from build123d import *

# Parameters (mm, degrees)
SKETCH1_R           = 2.159
SKETCH1_R_2         = 3.81
BOSS_EXTRUDE1_DEPTH = 1.5875
FILLET1_R           = 2.54
SKETCH2_W           = 5.08
SKETCH2_H           = 15.875
SKETCH2_W_2         = 2.54
SKETCH2_H_2         = 3.81
CUT_EXTRUDE1_DEPTH  = 1.5875
FILLET2_START       = -1
FILLET2_DEPTH       = 4
FILLET2_2_DEPTH     = 1.5875


with BuildPart() as part:
    # Sketch1 → Boss-Extrude1 (new body)
    with BuildSketch(Plane.XY):
        with BuildLine():
            Line((0, 38.1), (0, 0))
            Line((0, 0), (92.075, 0))
            Line((92.075, 0), (92.075, 38.1))
            ThreePointArc((92.075, 38.1), (81.75625, 48.41875), (71.4375, 38.1))
            Line((71.4375, 38.1), (71.4375, 9.271))
            Line((71.4375, 9.271), (20.6375, 9.271))
            Line((20.6375, 9.271), (20.6375, 38.1))
            ThreePointArc((20.6375, 38.1), (10.31875, 48.41875), (0, 38.1))
        make_face()
        with Locations((22.5425, 4.6355)):
            Circle(SKETCH1_R, mode=Mode.SUBTRACT)
        with Locations((69.5325, 4.6355)):
            Circle(SKETCH1_R, mode=Mode.SUBTRACT)
        with Locations((11.1125, 38.1)):
            Circle(SKETCH1_R_2, mode=Mode.SUBTRACT)
        with Locations((80.9625, 38.1)):
            Circle(SKETCH1_R_2, mode=Mode.SUBTRACT)
    extrude(amount=BOSS_EXTRUDE1_DEPTH)

    # Fillet1
    fillet1_edges = [part.edges().sort_by_distance(p)[0] for p in [
        (92.075, 0, 0.79375),
        (0, 0, 0.79375),
    ]]
    fillet(fillet1_edges, radius=FILLET1_R)

    # Sketch2 → Cut-Extrude1 (cut)
    with BuildSketch(Plane.XY.offset(1.5875)):
        with Locations((89.535, 22.2885)):
            Rectangle(SKETCH2_W, SKETCH2_H)
        with Locations((2.54, 22.2885)):
            Rectangle(SKETCH2_W, SKETCH2_H)
        with Locations((18.0975, 25.4)):
            Rectangle(SKETCH2_W_2, SKETCH2_H_2)
        with Locations((73.9775, 25.4)):
            Rectangle(SKETCH2_W_2, SKETCH2_H_2)
    extrude(amount=-CUT_EXTRUDE1_DEPTH, mode=Mode.SUBTRACT)

    # Fillet2: read off the stored shape, not the designer's step
    # Fillet2 outline → Fillet2 (cut)
    with BuildSketch(Plane.XY.offset(FILLET2_START)):
        with BuildLine():
            Line((92.075, 14.351), (89.535, 14.351))
            ThreePointArc((89.535, 14.351), (91.331051224, 13.607051224), (92.075, 11.811))
            Line((92.075, 11.811), (92.075, 14.351))
        make_face()
        with BuildLine():
            ThreePointArc((92.075, 32.766), (91.331051224, 30.969948776), (89.535, 30.226))
            Line((89.535, 30.226), (92.075, 30.226))
            Line((92.075, 30.226), (92.075, 32.766))
        make_face()
        with BuildLine():
            Line((0, 30.226), (2.54, 30.226))
            ThreePointArc((2.54, 30.226), (0.743948776, 30.969948776), (0, 32.766))
            Line((0, 32.766), (0, 30.226))
        make_face()
        with BuildLine():
            ThreePointArc((0, 11.811), (0.743948776, 13.607051224), (2.54, 14.351))
            Line((2.54, 14.351), (0, 14.351))
            Line((0, 14.351), (0, 11.811))
        make_face()
    extrude(amount=FILLET2_DEPTH, mode=Mode.SUBTRACT)

    # Fillet2 2 outline → Fillet2 2 (add)
    with BuildSketch(Plane.XY):
        with BuildLine():
            ThreePointArc((89.535, 14.351), (87.738948776, 15.094948776), (86.995, 16.891))
            Line((86.995, 16.891), (86.995, 14.351))
            Line((86.995, 14.351), (89.535, 14.351))
        make_face()
        with BuildLine():
            ThreePointArc((86.995, 27.686), (87.738948776, 29.482051224), (89.535, 30.226))
            Line((89.535, 30.226), (86.995, 30.226))
            Line((86.995, 30.226), (86.995, 27.686))
        make_face()
        with BuildLine():
            ThreePointArc((2.54, 30.226), (4.336051224, 29.482051224), (5.08, 27.686))
            Line((5.08, 27.686), (5.08, 30.226))
            Line((5.08, 30.226), (2.54, 30.226))
        make_face()
        with BuildLine():
            ThreePointArc((5.08, 16.891), (4.336051224, 15.094948776), (2.54, 14.351))
            Line((2.54, 14.351), (5.08, 14.351))
            Line((5.08, 14.351), (5.08, 16.891))
        make_face()
    extrude(amount=FILLET2_2_DEPTH)


solid = part.part
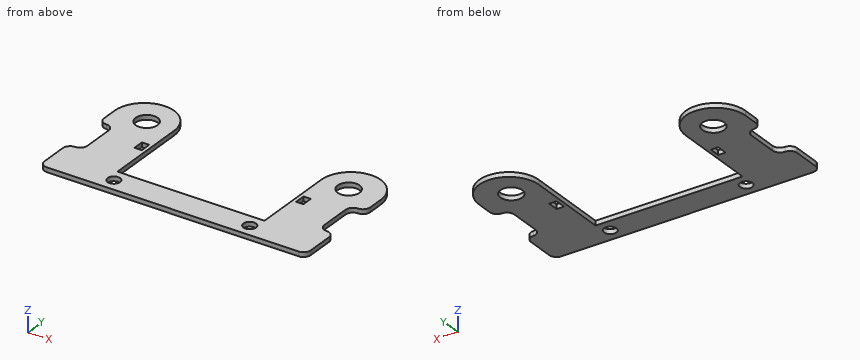
Verification items for the finished model (mm, model axes). Coordinates: 2 decimals unless noted, no trailing zeros. Order: outer loops, then holes, each group sorted by start corner. A loop starts at its lowest first (then second) coordinate and runs counter-clockwise, first axis right, second up. Notation, with made-up numbers: M 17.25,84.5 L 63.25,84.5 A29 cw 63.25,105.5 Z; hole C -22,38.25 d10. An arc over 180 degrees is marked long. One line per item, written item: value. Start each with the question number.
Item 1: Scan lines: probe 1 along X at (y, z) = (24, 0.75) (1 decimal); probe 2 along X at (y, z) = (4.5, 1.5) (3 decimals); probe 3 along X at (y, z) = (6.5, 0.25) (3 decimals). Record each from-to range of solid material in increasing order.
Item 2: Sectioned sample at C-C (z = 1.25). Count the separate pieces of the cut face and the enclosed holes in it, then the cut area to 3 significant figures.
Item 3: Sectioned sample at A-A (y = 18.5). Enter the section's corners in (x, z) (1 decimal), then the cut area to 3 significant figures.
Item 4: Sectioned sample at B-B (y = 3.5). Enter the section's corners in (x, z) (1 decimal), then the cut area to 3 significant figures.
Item 5: Gauge pin test, flat ends, axial feed: pin 1 (0.8 mm diameter, centred on y = 28, z = 1, fed in from -X); pin 2 (0.5 mm diameter, centred on y = 25, z = 1, fed in from -X); pin 3 (0.8 mm diameter, centred on y = 26, z = 1, fed in from +X) (3 decimals). Record the tip position at first contact, or that the pin passes through.
Item 6: Sectioned sample at D-D (y = 35.5). Enter the section's corners in (x, z) (1 decimal), then the cut area to 3 significant figures.
Conclusion:
1. probe 1: x = 5.1 to 16.8, 19.4 to 20.6, 71.4 to 72.7, 75.2 to 87
1. probe 2: x = 0 to 20.388, 24.697 to 67.378, 71.687 to 92.075
1. probe 3: x = 0 to 21.454, 23.631 to 68.444, 70.621 to 92.075
2. separate pieces: 1
2. enclosed holes: 6
2. area: 2,070 mm^2
3. outline: M 5.1,0 L 20.6,0 L 20.6,1.6 L 5.1,1.6 Z; M 71.4,0 L 87,0 L 87,1.6 L 71.4,1.6 Z
3. area: 49.4 mm^2
4. outline: M 0,0 L 20.7,0 L 20.7,1.6 L 0,1.6 Z; M 24.4,0 L 67.7,0 L 67.7,1.6 L 24.4,1.6 Z; M 71.4,0 L 92.1,0 L 92.1,1.6 L 71.4,1.6 Z
4. area: 135 mm^2
5. pin 1: stops at x = 4.98
5. pin 2: stops at x = 5.08
5. pin 3: stops at x = 86.995
6. outline: M 0,0 L 8.3,0 L 8.3,1.6 L 0,1.6 Z; M 13.9,0 L 20.6,0 L 20.6,1.6 L 13.9,1.6 Z; M 71.4,0 L 78.2,0 L 78.2,1.6 L 71.4,1.6 Z; M 83.7,0 L 92.1,0 L 92.1,1.6 L 83.7,1.6 Z
6. area: 47.8 mm^2
